Here's how the part is built. I have some questions about the finished solid (model axes, mm). Give positions to 0.01 mm unless a question says otherwise; leave off trailing zeros. Use one line per item in the form item = value.
from build123d import *

# Parameters (mm, degrees)
SKETCH1_W           = 154
SKETCH1_H           = 175
BOSS_EXTRUDE1_DEPTH = 1.6
FILLET1_R           = 3
SKETCH2_R           = 1.89865
CUT_EXTRUDE1_DEPTH  = 2.6
SKETCH3_R           = 1.63195
CUT_EXTRUDE2_DEPTH  = 2.6
SKETCH4_R           = 1.5
CUT_EXTRUDE3_DEPTH  = 2.6
SKETCH5_R           = 1.09
CUT_EXTRUDE4_DEPTH  = 2.6


with BuildPart() as part:
    # Sketch1 → Boss-Extrude1 (new body)
    with BuildSketch(Plane.XY):
        Rectangle(SKETCH1_W, SKETCH1_H)
    extrude(amount=BOSS_EXTRUDE1_DEPTH)

    # Fillet1
    fillet1_edges = [part.edges().sort_by_distance(p)[0] for p in [
        (77, -87.5, 0.8),
        (-77, -87.5, 0.8),
        (-77, 87.5, 0.8),
        (77, 87.5, 0.8),
    ]]
    fillet(fillet1_edges, radius=FILLET1_R)

    # Sketch2 → Cut-Extrude1 (cut, through all)
    with BuildSketch(Plane.XY.offset(1.6)):
        with Locations((-70.612, 80.137)):
            Circle(SKETCH2_R)
        with Locations((70.612, 80.137)):
            Circle(SKETCH2_R)
        with Locations((70.612, -80.137)):
            Circle(SKETCH2_R)
        with Locations((-70.612, -80.137)):
            Circle(SKETCH2_R)
    extrude(amount=-CUT_EXTRUDE1_DEPTH, mode=Mode.SUBTRACT)

    # Sketch3 → Cut-Extrude2 (cut, through all)
    with BuildSketch(Plane.XY.offset(1.6)):
        with Locations((1.460377772, 64.310456987)):
            Circle(SKETCH3_R)
        with Locations((37.909377772, 64.310456987)):
            Circle(SKETCH3_R)
        with Locations((37.909377772, 22.400456987)):
            Circle(SKETCH3_R)
        with Locations((1.460377772, 22.400456987)):
            Circle(SKETCH3_R)
        with Locations((33.813625676, 11.150933339)):
            Circle(SKETCH3_R)
        with Locations((70.262625674, 11.150933339)):
            Circle(SKETCH3_R)
        with Locations((70.262625674, -30.759066661)):
            Circle(SKETCH3_R)
        with Locations((33.813625676, -30.759066661)):
            Circle(SKETCH3_R)
        with Locations((1.126771482, -38.187714501)):
            Circle(SKETCH3_R)
        with Locations((37.575771481, -38.187714501)):
            Circle(SKETCH3_R)
        with Locations((37.575771481, -80.097714501)):
            Circle(SKETCH3_R)
        with Locations((1.126771482, -80.097714501)):
            Circle(SKETCH3_R)
        with Locations((-31.190042853, 11.891013056)):
            Circle(SKETCH3_R)
        with Locations((5.258957145, 11.891013056)):
            Circle(SKETCH3_R)
        with Locations((5.258957145, -30.018986944)):
            Circle(SKETCH3_R)
        with Locations((-31.190042853, -30.018986944)):
            Circle(SKETCH3_R)
        with Locations((-61.163271416, -36.707555066)):
            Circle(SKETCH3_R)
        with Locations((-24.714271417, -36.707555066)):
            Circle(SKETCH3_R)
        with Locations((-24.714271417, -78.617555066)):
            Circle(SKETCH3_R)
        with Locations((-61.163271416, -78.617555066)):
            Circle(SKETCH3_R)
    extrude(amount=-CUT_EXTRUDE2_DEPTH, mode=Mode.SUBTRACT)

    # Sketch4 → Cut-Extrude3 (cut, through all)
    with BuildSketch(Plane.XY.offset(1.6)):
        with Locations((12.986023067, 34.581675178)):
            Circle(SKETCH4_R)
        with Locations((61.986023067, 34.581675178)):
            Circle(SKETCH4_R)
        with Locations((61.986023067, -23.418324822)):
            Circle(SKETCH4_R)
        with Locations((12.986023067, -23.418324822)):
            Circle(SKETCH4_R)
    extrude(amount=-CUT_EXTRUDE3_DEPTH, mode=Mode.SUBTRACT)

    # Sketch5 → Cut-Extrude4 (cut, through all)
    with BuildSketch(Plane(origin=(0, 0, 0), x_dir=(-1, 0, 0), z_dir=(0, 0, -1))):
        with Locations((41.518941969, 72.631735316)):
            Circle(SKETCH5_R)
        with Locations((57.518941969, 59.131735316)):
            Circle(SKETCH5_R)
        with Locations((18.301790213, -77.528250676)):
            Circle(SKETCH5_R)
        with Locations((5.101790213, -64.328250676)):
            Circle(SKETCH5_R)
    extrude(amount=-CUT_EXTRUDE4_DEPTH, mode=Mode.SUBTRACT)


solid = part.part
(1) If I drill on probe 1 along X at (y, z) = (-64.5, 1.25); probe 2 along Y at (x, z) = (-69.5, 1.25); probe 3 along Y at (x, z) = (-24, 1.05), over which ranges is the centre line in solid material (lowest first)?
Geometry says:
probe_1 = -77 to -6.18, -4.03 to 77
probe_2 = -87.5 to -81.68, -78.6 to 78.6, 81.68 to 87.5
probe_3 = -87.5 to -80.08, -77.15 to -38.17, -35.24 to 87.5
(2) Thinking about a two-plate mould opening in X: for faces 1 (the cylindrical face through (69.105, 78.982, 0.811)), 2 (the flat face through (-1, 1, 1.6)), 3 (the cylindrical face through (70.365, -78.255, 0.811)), which applies, pulls with the +X half, pulls with the -X half, needs draft (parallel to the pull), parting line crosses it, or undercut?
Geometry says:
face_1 = undercut
face_2 = needs draft
face_3 = undercut
(3) For P1, Ø8, axis at x = -50, y = -61, coming from the -Z side; P2, Ø1.7, axis at x = -57.52, y = 59.13, coming from the -Z side, each with a flat end and sliding along its axis, tell me the tip position at first contact or that it passes through.
Geometry says:
P1 = 0
P2 = through
